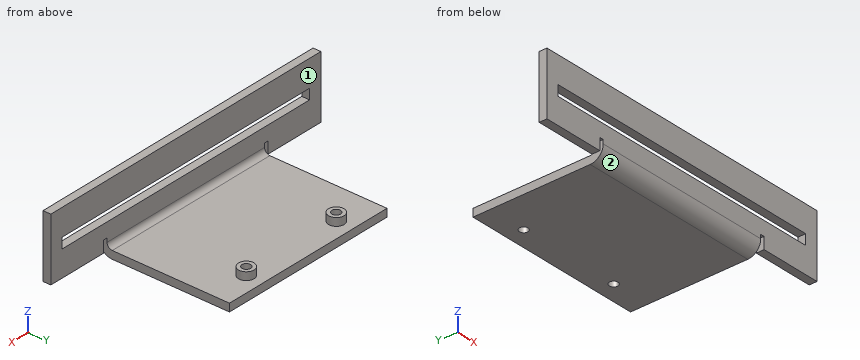
from build123d import *

# Parameters (mm, degrees)
SM_BASE_FLANGE_2_DEPTH            = 3
SM_EDGE_FLANGE_2_STRIP_W          = 16
SM_EDGE_FLANGE_2_STRIP_H          = 3
SM_EDGE_FLANGE_2_STRIP_CUT_DEPTH  = 70
SM_EDGE_FLANGE_2_RELIEF_W         = 17.5
SM_EDGE_FLANGE_2_RELIEF_H         = 1.5
SM_EDGE_FLANGE_2_RELIEF_CUT_DEPTH = 3
SM_EDGE_FLANGE_2_DEPTH            = 70
SKETCH_21_W                       = 110
SKETCH_21_H                       = 4
CUT_EXTRUDE_1_DEPTH               = 30
SKETCH_23_R                       = 3
EXTRUDE_1_DEPTH                   = 3
SKETCH_24_R                       = 1.65
CUT_EXTRUDE_2_DEPTH               = 6


# Sheet-metal steps are written as plain solids
with BuildPart() as part:
    # 草图15 → 基体-法兰2 (new body)
    with BuildSketch(Plane(origin=(0, 0, 0), x_dir=(1, 0, 0), z_dir=(0, 1, 0))):
        Polygon((0, -41.752065), (120, -41.752065), (120, -17.652065), (95, -17.652065), (95, -15.652065), (25, -15.652065), (25, -17.652065), (0, -17.652065), align=None)
    extrude(amount=-SM_BASE_FLANGE_2_DEPTH)

    # 边线-法兰2 strip (across the edge) → 边线-法兰2 strip cut (cut)
    with BuildSketch(Plane(origin=(95, 0, 15.652065), x_dir=(0, 0, 1), z_dir=(-1, 0, 0))):
        with Locations((-3, -1.5)):
            Rectangle(SM_EDGE_FLANGE_2_STRIP_W, SM_EDGE_FLANGE_2_STRIP_H)
    extrude(amount=SM_EDGE_FLANGE_2_STRIP_CUT_DEPTH, mode=Mode.SUBTRACT)

    # 边线-法兰2 relief (on the sheet) → 边线-法兰2 relief cut (cut)
    with BuildSketch(Plane(origin=(95, 0, 20.652065), x_dir=(0, 0, 1), z_dir=(0, 1, 0))):
        with Locations((-7.25, 0.75)):
            Rectangle(SM_EDGE_FLANGE_2_RELIEF_W, SM_EDGE_FLANGE_2_RELIEF_H)
        with Locations((-7.25, -70.75)):
            Rectangle(SM_EDGE_FLANGE_2_RELIEF_W, SM_EDGE_FLANGE_2_RELIEF_H)
    extrude(amount=-SM_EDGE_FLANGE_2_RELIEF_CUT_DEPTH, mode=Mode.SUBTRACT)

    # 边线-法兰2 section (across the edge) → 边线-法兰2 (add)
    with BuildSketch(Plane(origin=(95, 0, 15.652065), x_dir=(0, 0, 1), z_dir=(-1, 0, 0))):
        with BuildLine():
            Line((0, 2), (0, 47))
            Line((0, 47), (3, 47))
            Line((3, 47), (3, 2))
            ThreePointArc((3, 2), (3.585786438, 0.585786438), (5, 0))
            Line((5, 0), (5, -3))
            ThreePointArc((5, -3), (1.464466094, -1.535533906), (0, 2))
        make_face()
    extrude(amount=SM_EDGE_FLANGE_2_DEPTH)

    # 草图21 → 切除-拉伸1 (cut)
    with BuildSketch(Plane(origin=(0, 0, 0), x_dir=(1, 0, 0), z_dir=(0, 1, 0))):
        with Locations((60, -29.58826484)):
            Rectangle(SKETCH_21_W, SKETCH_21_H)
    extrude(amount=-CUT_EXTRUDE_1_DEPTH, mode=Mode.SUBTRACT)

    # 草图23 → 凸台-拉伸1 (add)
    with BuildSketch(Plane.XY.offset(18.652065)):
        with Locations((40, 40.5)):
            Circle(SKETCH_23_R)
        with Locations(Location((80, 40.5, 0), (0, 0, 180))):
            Circle(SKETCH_23_R)
    extrude(amount=EXTRUDE_1_DEPTH)

    # 草图24 → 切除-拉伸2 (cut)
    with BuildSketch(Plane.XY.offset(21.652065)):
        with Locations((40, 40.5)):
            Circle(SKETCH_24_R)
        with Locations((80, 40.5)):
            Circle(SKETCH_24_R)
    extrude(amount=-CUT_EXTRUDE_2_DEPTH, mode=Mode.SUBTRACT)


solid = part.part
Can you work these out from the model? Positions are in its coordinate system, mm. Face numbers are marked on the shaded views. Coordinates: 2 decimals unless noted, no trailing zeros. Write each loop counter-clockwise with the first axis right and the second up, starting at its lowest first coordinate (ties: lowest second). Pieces come first, ordered by that corner, then holes. Notation, with made-up numbers: (41, 10.25) -> (50, 10.25) arc R16 ccw to (50, 20.25) -> close; hole circle Ø2 at (64.25, 6.5). An arc over 180 degrees is marked (long way). Write item = value, one per line.
(1) Imagine slicing it at A-A (x = 72.5). Please give me the cut outline in (y, z), and give its area (3 significant figures).
Verdict:
outline = (-3, 20.65) arc R5 ccw to (2, 15.65) -> (47, 15.65) -> (47, 18.65) -> (2, 18.65) arc R2 cw to (0, 20.65) -> (0, 27.59) -> (-3, 27.59) -> close; (-3, 31.59) -> (0, 31.59) -> (0, 41.75) -> (-3, 41.75) -> close
area = 203 mm^2
(2) Imagine slicing it at D-D (y = 4.5). Please give me the cut outline in (x, z).
Verdict:
outline = (25, 15.65) -> (95, 15.65) -> (95, 18.65) -> (25, 18.65) -> close
(3) Imagine slicing it at B-B (y = 40.5). Please give me the cut outline in (x, z).
Verdict:
outline = (25, 15.65) -> (38.35, 15.65) -> (38.35, 21.65) -> (37, 21.65) -> (37, 18.65) -> (25, 18.65) -> close; (41.65, 15.65) -> (78.35, 15.65) -> (78.35, 21.65) -> (77, 21.65) -> (77, 18.65) -> (43, 18.65) -> (43, 21.65) -> (41.65, 21.65) -> close; (81.65, 15.65) -> (95, 15.65) -> (95, 18.65) -> (83, 18.65) -> (83, 21.65) -> (81.65, 21.65) -> close
(4) Thinking about a two-plate mould opening in X: for the marked faces 1 and 2, which applies, +X half, -X half, draft (parallel to the pull), parting line (faces both ways), or undercut?
Verdict:
face_1 = draft
face_2 = undercut
(5) Imagine slicing it at C-C (z = 37.25). Please give me the cut outline in (x, y).
Verdict:
outline = (0, -3) -> (120, -3) -> (120, 0) -> (0, 0) -> close
(6) For pin 1 (3 mm diameter, centred on x = 41, y = 39.5, fed in from +Z); pin 2 (0.8 mm diameter, centred on x = 95.5, y = -1.5, fed in from -Z); pin 3 (10 mm diameter, centred on y = 15, z = 23.5, fed in from +X); pin 4 (0.9 mm diameter, centred on y = -1, z = 30, fed in from -X), each with a flat end and sliding along its axis, tell me the tip position at first contact or that it passes through.
Verdict:
pin_1 = 21.65
pin_2 = 22.15
pin_3 = 95
pin_4 = 0
(7) If I drill on probe 1 along Z at (x, y) = (69.5, 28.5); probe 2 along Y at (x, z) = (80, 18.5); probe 3 along Y at (x, z) = (43, 38.75), over which ranges is the centre line in solid material (lowest first)?
Verdict:
probe_1 = 15.65 to 18.65
probe_2 = -2.51 to 38.85, 42.15 to 47
probe_3 = -3 to 0
